Autodesk Fusion 360 part; units mm, degrees
sketch "Sketch1" plane through (0, 0, 0) normal (0, 1, 0) x (1, 0, 0)
  line L0 (0, 0) -> (0, -188.5)
  line L1 (0, 0) -> (-0.6248, 0)
  line L2 (-0.6248, 0) -> (-2.1248, 0)
  line L3 (-2.1248, 0) -> (-2.1248, -188.5)
  line L4 (-2.1248, -188.5) -> (0, -188.5)
  dimension "d1" = 188.5
  dimension "d2" = 1.5
revolve "Revolve1" add sketch "Sketch1" angle 360 about axis through (0, 0, 0) along (0, 0, 1)
sketch "Sketch2" plane through (0, 0, 0) normal (0, 0, -1) x (1, 0, 0)
  circle A0 centre (0, 0) radius 2.1248
  line L0 (0, 0.5) -> (-3, 0.5)
  line L1 (0, 0.5) -> (3.7205, 0.5)
  line L2 (3.7205, -0.5) -> (-3, -0.5)
  line L3 (0, 0.5) -> (5, 0.5)
  line L4 (5, 0.5) -> (5, -0.5)
  line L5 (5, -0.5) -> (-5, -0.5)
  line L6 (-5, -0.5) -> (-5, 0.5)
  line L7 (-5, 0.5) -> (-5.1, 0.5)
  line L8 (-5, 0.5) -> (5, 0.5)
  dimension "d4" = 0.5
extrude "Extrude2" add sketch "Sketch2" against normal blind 14 contours A0 L0 L2 L5 L6 L8
extrude "Extrude1" add sketch "Sketch2" against normal blind 14 contours A0 L1 L2 L3 L4 L5 L8
hole "Hole1" at (0, 0, 188.5) direction (0, 0, -1) diameter 2.529 depth 25 tip angle 118
Here's how the part is built. I have some questions about the finished solid (model axes, mm). A direction names the side the tool comes from. Give positions to 0.01 mm unless a question says otherwise; leave off trailing zeros. Write each loop counter-clockwise with the first axis right and the second up, starting at its lowest first coordinate (ties: lowest second). Pieces come first, ordered by that corner, then holes.
(1) If I drill on L1, parallel to Y at x = 0, z = 176.5; L2, parallel to Y at x = -0.25, z = 168.5, over which ranges is the centre line in solid material (lowest first)?
Output values:
L1: y = -2.12 to -1.26, 1.26 to 2.12
L2: y = -2.11 to -1.24, 1.24 to 2.11
(2) Imagine slicing it at A-A, the plane z = 52.5. Write out the boundary of the cut face in (x, y).
Output values:
outline: circle Ø4.25 at (0, 0)
(3) On a 3-axis mill with a long thin cutter (end or side, diameter ignored), from which of +Z, -Z, +X, -X, +Y, -Y can I reach the whole of each face in a straight line? I mean faces 1 (the face through (4, 0.5, 7)), 2 (the face through (4, -0.5, 7)), 3 (the face through (-4, 0.5, 7)), 4 (the face through (-4, -0.5, 7)). Say none if no direction works.
Output values:
face 1: +Z, -Z, +X, +Y
face 2: +Z, -Z, +X, -Y
face 3: +Z, -Z, -X, +Y
face 4: +Z, -Z, -X, -Y
(4) Will these pins go through, and if not, where does the flat tip stop? pin 1 (4 mm diameter, centred on x = -3.5, z = 144, fed in from +Y); pin 2 (0.8 mm diameter, centred on x = 4, y = 0, fed in from +Z); pin 3 (2.5 mm diameter, centred on x = 3, z = 8.5, fed in from -Y).
Output values:
pin 1: stops at y = 1.5
pin 2: stops at z = 14
pin 3: stops at y = -1.21
